```python
from build123d import *

# Parameters (mm, degrees)
CROQUIS1_W              = 120
CROQUIS1_H              = 10
CROQUIS1_R              = 2.1
SALIENTE_EXTRUIR1_DEPTH = 3
CROQUIS2_R              = 2.1
CORTAR_EXTRUIR1_DEPTH   = 3


with BuildPart() as part:
    # Croquis1 → Saliente-Extruir1 (new body)
    with BuildSketch(Plane(origin=(0, 0, 0), x_dir=(1, 0, 0), z_dir=(0, 1, 0))):
        Rectangle(CROQUIS1_W, CROQUIS1_H)
        with Locations(Location((-55, 0, 0), (0, 0, 270))):
            Circle(CROQUIS1_R, mode=Mode.SUBTRACT)
        with Locations(Location((-45, 0, 0), (0, 0, 270))):
            Circle(CROQUIS1_R, mode=Mode.SUBTRACT)
        with Locations(Location((-35, 0, 0), (0, 0, 270))):
            Circle(CROQUIS1_R, mode=Mode.SUBTRACT)
        with Locations(Location((-25, 0, 0), (0, 0, 270))):
            Circle(CROQUIS1_R, mode=Mode.SUBTRACT)
    extrude(amount=SALIENTE_EXTRUIR1_DEPTH)

    # Croquis2 → Cortar-Extruir1 (cut)
    with BuildSketch(Plane(origin=(0, 3, 0), x_dir=(1, 0, 0), z_dir=(0, 1, 0))):
        with Locations(Location((55, 0, 0), (0, 0, 270))):
            Circle(CROQUIS2_R)
        with Locations(Location((45, 0, 0), (0, 0, 270))):
            Circle(CROQUIS2_R)
    extrude(amount=-CORTAR_EXTRUIR1_DEPTH, mode=Mode.SUBTRACT)


solid = part.part
```
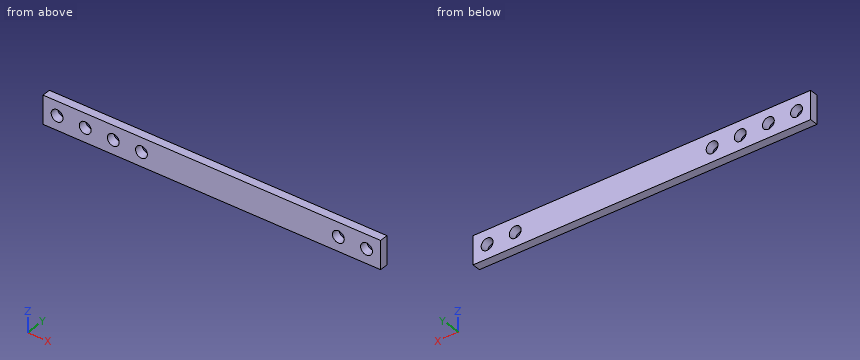
CAD build for the part. Positions are in the model's coordinates, mm. Round coordinates to 2 decimals unless told otherwise and drop trailing zeros. Order: outer loops, then holes, each group sorted by start corner. A loop starts at its lowest first (then second) coordinate and runs counter-clockwise, first axis right, second up.
Item 1: Probe line 1 along Z through (x, y) = (54.5, 2.6). List the from-to ranges inside material, lowest first.
Item 2: Saw through at B-B on y = 0.8. Write the cut outline in (x, z), then the cut area to 3 significant figures.
Item 3: Pin check, flat tip, straight feed: pin 1 (2.5 mm diameter, centred on x = -55, z = 0, fed in from +Y). Stop position of the tip, or through.
Item 4: Saw through at A-A on x = -45. Write the cut outline in (y, z).
Item 5: Saw through at C-C on z = -1. Write the cut outline in (x, y), then the cut area to 3 significant figures.
Reported:
1. line 1: z = -5 to -2.04, 2.04 to 5
2. outline: (-60, -5) - (60, -5) - (60, 5) - (-60, 5) - close; hole circle Ø4.2 at (-55, 0); hole circle Ø4.2 at (-45, 0); hole circle Ø4.2 at (-35, 0); hole circle Ø4.2 at (-25, 0); hole circle Ø4.2 at (45, 0); hole circle Ø4.2 at (55, 0)
2. area: 1,120 mm2
3. pin 1: passes through
4. outline: (0, -5) - (3, -5) - (3, -2.1) - (0, -2.1) - close; (0, 2.1) - (3, 2.1) - (3, 5) - (0, 5) - close
5. outline: (-60, 0) - (-56.85, 0) - (-56.85, 3) - (-60, 3) - close; (-53.15, 0) - (-46.85, 0) - (-46.85, 3) - (-53.15, 3) - close; (-43.15, 0) - (-36.85, 0) - (-36.85, 3) - (-43.15, 3) - close; (-33.15, 0) - (-26.85, 0) - (-26.85, 3) - (-33.15, 3) - close; (-23.15, 0) - (43.15, 0) - (43.15, 3) - (-23.15, 3) - close; (46.85, 0) - (53.15, 0) - (53.15, 3) - (46.85, 3) - close; (56.85, 0) - (60, 0) - (60, 3) - (56.85, 3) - close
5. area: 294 mm2
